from build123d import *

# Parameters (mm, degrees)
ESQUISSE3_R             = 1.25
ENL_V_MAT_EXTRU_1_DEPTH = 6


with BuildPart() as part:
    # Esquisse1 → Révolution1 (revolve)
    with BuildSketch(Plane.XY):
        Polygon((0, 0), (0, 1), (-10, 1), (-10, 2.5), (-16, 2.5), (-16, 0), align=None)
    revolve(axis=Axis((0, -2, 0), (-1, 0, 0)))

    # Esquisse3 → Enlèv. mat.-Extru.1 (cut)
    with BuildSketch(Plane(origin=(0, 3, 0), x_dir=(-1, 0, 0), z_dir=(0, 1, 0))):
        with Locations((13, 0)):
            Circle(ESQUISSE3_R)
    extrude(amount=-ENL_V_MAT_EXTRU_1_DEPTH, mode=Mode.SUBTRACT)


solid = part.part
CAD build for the part. Positions are in the model's coordinates, mm. A direction names the side the tool comes from. Round coordinates to 2 decimals unless told otherwise and drop trailing zeros. Write each loop counter-clockwise with the first axis right and the second up, starting at its lowest first coordinate (ties: lowest second). Pieces come first, ordered by that corner, then holes.
(1) Slice it at D-D, the plane z = -1.75. Write the cut outline in (x, y), and give its area (3 significant figures).
(2) Slice it at A-A, the plane y = -2. Write the cut outline in (x, z), and give its area (3 significant figures).
(3) Mould opens along Z. For faces 3 (the face through (-14.155, 1.051, -0.479)), 4 (the face through (-13.04, -2.59, -4.46)), 5 (the face through (0, -3, 2)) say: pulls with the +Z half, pulls with the -Z half, needs draft (parallel to the pull), parting line crosses it, or undercut.
(4) Slice it at C-C, the plane x = -4.5. Write the cut outline in (y, z).
(5) Probe line 1 along Z through (x, y) = (-3.25, -2); line 2 along Z through (x, y) = (-12.5, -2); line 3 along Y through (x, z) = (-9, 0). List the from-to ranges inside material, lowest first.
(6) 3-axis set-ups, long thin cutter, end or side, ignore diameter. For faces 1 (the face through (-5.1, -4.4, 1.8)), 2 (the face through (-8, -4, 0)): which of +Z, -Z, +X, -X, +Y, -Y reach the whole face in a straight line?
(7) Slice it at B-B, the plane z = 0. Write the cut outline in (x, y), and give its area (4 significant figures).
(8) Drop flat-ended pins along their axis: P1, Ø1, axis at y = 1, z = 2, coming from the +X side; P2, Ø3, axis at y = -2, z = 0, coming from the +X side; P3, Ø1, axis at x = -6.5, z = -3, coming from the -Y side. Give the stop position or say it passes through.
From the geometry:
1. outline: (-16, -6.15) - (-10, -6.15) - (-10, -4.44) - (0, -4.44) - (0, -2.97) - (-16, -2.97) - close; (-16, -1.03) - (0, -1.03) - (0, 0.44) - (-10, 0.44) - (-10, 2.15) - (-16, 2.15) - close
1. area: 67.5 mm2
2. outline: (-16, -4.5) - (-10, -4.5) - (-10, -3) - (0, -3) - (0, -2) - (-16, -2) - close; (-16, 2) - (0, 2) - (0, 3) - (-10, 3) - (-10, 4.5) - (-16, 4.5) - close
2. area: 50.0 mm2
3. face 3: undercut
3. face 4: parting line crosses it
3. face 5: needs draft
4. outline: circle Ø6 at (-2, 0); hole circle Ø4 at (-2, 0)
5. line 1: z = -3 to -2, 2 to 3
5. line 2: z = -4.5 to -2, 2 to 4.5
5. line 3: y = -5 to -4, 0 to 1
6. face 1: +X
6. face 2: +X, -X
7. outline: (-16, -6.5) - (-10, -6.5) - (-10, -5) - (0, -5) - (0, -4) - (-16, -4) - close; (-16, 0) - (-14.25, 0) - (-14.25, 2.5) - (-16, 2.5) - close; (-11.75, 0) - (0, 0) - (0, 1) - (-10, 1) - (-10, 2.5) - (-11.75, 2.5) - close
7. area: 43.75 mm2
8. P1: stops at x = -10
8. P2: passes through
8. P3: stops at y = -3.66
